Design review of the part built by this model. Coordinates are the model's own, in mm. A direction names the side the tool comes from. Give positions to 0.01 mm unless a question says otherwise; leave off trailing zeros. Loops run counter-clockwise (first coordinate to the right, second up) from the corner with the lowest first, then second, coordinate; pieces in that order, holes last.
from build123d import *

# Parameters (mm, degrees)
ENL_V_MAT_EXTRU_1_DEPTH      = 59.776504379
R_P_TITION_CIRCULAIRE1_COUNT = 6


with BuildPart() as part:
    # Esquisse1 → R_volution1 (revolve)
    with BuildSketch(Plane.XY, mode=Mode.PRIVATE) as r_volution1_sk:
        with BuildLine():
            Line((-4, 12), (-4, 0))
            Line((-4, 0), (-13, 0))
            Line((-13, 0), (-13, 1.5))
            Line((-13, 1.5), (-18, 1.5))
            ThreePointArc((-18, 1.5), (-20.050252532, 6.449747468), (-25, 8.5))
            Line((-25, 8.5), (-38, 8.5))
            ThreePointArc((-38, 8.5), (-39.207317246, 14), (-38, 19.5))
            Line((-38, 19.5), (-26.383086274, 19.5))
            Line((-26.383086274, 19.5), (-17, 12))
            Line((-17, 12), (-4, 12))
        make_face()
    revolve(r_volution1_sk.sketch.rotate(Axis((0, 0, 0), (0, 1, 0)), 270), axis=Axis((0, 0, 0), (0, 1, 0)))

    # Esquisse2 → Enl_v. mat.-Extru.1 (cut, through all)
    with BuildSketch(Plane(origin=(0, 19.5, 0), x_dir=(1, 0, 0), z_dir=(0, 1, 0))):
        with BuildLine():
            Line((-18.717027808, -39.248205418), (0, -70))
            Line((0, -70), (18.717027808, -39.248205418))
            ThreePointArc((18.717027808, -39.248205418), (0, -34), (-18.717027808, -39.248205418))
        make_face()
    enl_v_mat_extru_1 = extrude(amount=-ENL_V_MAT_EXTRU_1_DEPTH, mode=Mode.SUBTRACT)

    # R_p_tition circulaire1: Enl_v. mat.-Extru.1 ×6 about axis
    r_p_tition_circulaire1_axis = Axis((0, 0, 0), (0, 1, 0))
    for i in range(1, R_P_TITION_CIRCULAIRE1_COUNT):
        add(enl_v_mat_extru_1.rotate(r_p_tition_circulaire1_axis, i * 360 / R_P_TITION_CIRCULAIRE1_COUNT), mode=Mode.SUBTRACT)


solid = part.part
Q1. Draft analysis for pull direction X (two halves, no side actions). For faces 1 (the face through (0, 14, 34)), 2 (the face through (29.347, 14.077, -17.171)), 3 (the face through (7.91, 0.76, 10.316)), state which applies: pulls with the +X half, pulls with the -X half, needs draft (parallel to the pull), parting line crosses it, or undercut.
Results:
face 1: undercut
face 2: pulls with the +X half
face 3: parting line crosses it
Q2. Tool access review of faces 4 (the face through (-9.4, 1.5, 9.2)), 5 (the face through (4, 12, -4)), 6 (the face through (-29.347, 14.077, 17.171)): name each direction out of +Z, -Z, +X, -X, +Y, -Y from which nothing blocks a thin tool from reaching the whole face with its end or side.
Results:
face 4: -Y
face 5: +Y
face 6: +Z, -X, +Y, -Y
Q3. Wall thickness on line 1 (Y direction, x = 30.5, z = 1.5); line 2 (Y direction, x = -8.5, z = -14.5); line 3 (Z direction, x = 1, y = 9): over which ranges is each line inside the solid? List them lowest first.
Results:
line 1: y = 8.5 to 19.5
line 2: y = 1.5 to 12
line 3: z = -34.01 to -3.87, 3.87 to 34.01
Q4. Take a section at C-C (y = 14.75). Give the boundary of the cut face in (x, z).
Results:
outline: (-38.65, -6.49) arc R36 cw to (-24.94, -30.22) arc R39.19 ccw to (-13.71, -36.71) arc R36 cw to (13.71, -36.71) arc R39.19 ccw to (24.94, -30.22) arc R36 cw to (38.65, -6.49) arc R39.19 ccw to (38.65, 6.49) arc R36 cw to (24.94, 30.22) arc R39.19 ccw to (13.71, 36.71) arc R36 cw to (-13.71, 36.71) arc R39.19 ccw to (-24.94, 30.22) arc R36 cw to (-38.65, 6.49) arc R39.19 ccw to start; hole circle Ø40.88 at (0, 0)
Q5. Take a section at B-B (z = 0). Give the boundary of the cut face in (x, y).
Results:
outline: (-38, 8.5) - (-25, 8.5) arc R7 cw to (-18, 1.5) - (-13, 1.5) - (-13, 0) - (-4, 0) - (-4, 12) - (-17, 12) - (-26.38, 19.5) - (-38, 19.5) arc R13.13 ccw to start; (4, 0) - (13, 0) - (13, 1.5) - (18, 1.5) arc R7 cw to (25, 8.5) - (38, 8.5) arc R13.13 ccw to (38, 19.5) - (26.38, 19.5) - (17, 12) - (4, 12) - close
Q6. Take a section at D-D (y = 10). Give the boundary of the cut face in (x, z).
Results:
outline: (-37.93, -7.05) arc R36 cw to (-25.07, -29.33) arc R38.58 ccw to (-12.86, -36.38) arc R36 cw to (12.86, -36.38) arc R38.58 ccw to (25.07, -29.33) arc R36 cw to (37.93, -7.05) arc R38.58 ccw to (37.93, 7.05) arc R36 cw to (25.07, 29.33) arc R38.58 ccw to (12.86, 36.38) arc R36 cw to (-12.86, 36.38) arc R38.58 ccw to (-25.07, 29.33) arc R36 cw to (-37.93, 7.05) arc R38.58 ccw to start; hole circle Ø8 at (0, 0)
Q7. Take a section at A-A (x = 0). Give the boundary of the cut face in (y, z).
Results:
outline: (0, -13) - (1.5, -13) - (1.5, -18) arc R7 cw to (8.5, -25) - (8.5, -34) - (19.5, -34) - (19.5, -26.38) - (12, -17) - (12, -4) - (0, -4) - close; (0, 4) - (12, 4) - (12, 17) - (19.5, 26.38) - (19.5, 34) - (8.5, 34) - (8.5, 25) arc R7 cw to (1.5, 18) - (1.5, 13) - (0, 13) - close
Q8. Insertion check: pin 1 (2 mm diameter, centred on x = 0.5, z = 6.5, fed in from +Y); pin 2 (1.5 mm diameter, centred on x = -15.5, z = -14, fed in from -Y); pin 3 (4 mm diameter, centred on y = 3.5, z = 2, fed in from -X). Each pin has a flat end and moves straight along its axis. Give the tip position at first contact, or say it passes through.
Results:
pin 1: stops at y = 12
pin 2: stops at y = 6.53
pin 3: stops at x = -19.16
